For this review, take the finished solid that the model builds, in its own axes (mm). Face numbers are marked on the shaded views. A direction names the side the tool comes from. Coordinates: 2 decimals unless noted, no trailing zeros. Loops run counter-clockwise (first coordinate to the right, second up) from the corner with the lowest first, then second, coordinate; pieces in that order, holes last. Notation, with made-up numbers: (-24.75, 16.5) -> (-1.75, 16.5) arc R25 cw to (-1.75, 40.5) -> close; hole circle Ø9 at (40, 59). An arc over 180 degrees is marked (long way). Use a Markdown table: item, result.
from build123d import *

# Parameters (mm, degrees)
F0_W     = 38.1
F0_H     = 38.1
F1_DEPTH = 9.525
F2_SIZE  = 6.35
F3_W     = 38.1
F3_H     = 12.7
F4_DEPTH = 3.175


# Not quite as in the source:
# - a feature of the source that left no trace in its solid (it failed there, or was rolled back) is left out


with BuildPart() as f1:
    # F0 (on Top) → F1 (new body)
    with BuildSketch(Plane.XY):
        Rectangle(F0_W, F0_H)
    extrude(amount=F1_DEPTH)

    # F2
    f2_edges = [f1.edges().sort_by_distance(p)[0] for p in [
        (0, -19.05, 9.525),
    ]]
    chamfer(f2_edges, length=F2_SIZE)

    # F3 (on face) → F4 (join)
    with BuildSketch(Plane(origin=(0, 0, 0), x_dir=(1, 0, 0), z_dir=(0, 0, -1))):
        with Locations((0, 12.7)):
            Rectangle(F3_W, F3_H)
    extrude(amount=F4_DEPTH)


solid = f1.part
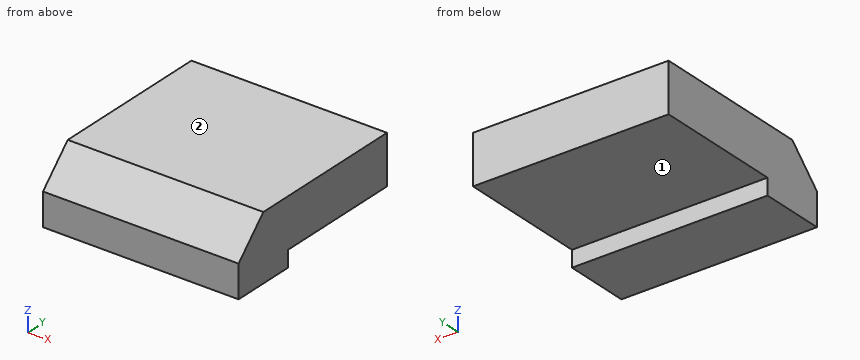
(1) Take a section at A-A on x = -15. Write out the cut boundary in (y, z) (3 decimals), plus the area to 3 significant figures.
Found:
| item | result |
|---|---|
| outline | (-19.05, -3.175) -> (-6.35, -3.175) -> (-6.35, 0) -> (19.05, 0) -> (19.05, 9.525) -> (-12.7, 9.525) -> (-19.05, 3.175) -> close |
| area | 383 mm^2 |
(2) For line 1 along Y through (x, z) = (-3, -1.5); line 2 along Z through (x, y) = (-7, -1) (3 decimals); line 3 along Y through (x, z) = (-12, 7.5) (3 decimals), list the stretches that pass through material, from the lowest coordinate up.
Found:
| item | result |
|---|---|
| line 1 | y = -19.05 to -6.35 |
| line 2 | z = 0 to 9.525 |
| line 3 | y = -14.725 to 19.05 |
(3) Take a section at B-B on y = 0.5. Write out the cut boundary in (x, z) (3 decimals).
Found:
| item | result |
|---|---|
| outline | (-19.05, 0) -> (19.05, 0) -> (19.05, 9.525) -> (-19.05, 9.525) -> close |
(4) For the marked faces 1 and 2, list the 3-axis set-ups (+Z, -Z, +X, -X, +Y, -Y) from which the entire face can be reached by the end or side of a thin tool; tool diameter is ignored.
Found:
| item | result |
|---|---|
| face 1 | -Z, +X, -X, +Y |
| face 2 | +Z, +X, -X, +Y, -Y |
(5) Take a section at C-C on z = 6.75. Write out the cut boundary in (x, y) (3 decimals).
Found:
| item | result |
|---|---|
| outline | (-19.05, -15.475) -> (19.05, -15.475) -> (19.05, 19.05) -> (-19.05, 19.05) -> close |
(6) For pin 1 Ø1 at (x, z) = (-1.5, -1) entering from +Y; pin 2 Ø6 at (x, y) = (-0.5, 11.5) entering from -Z, all flat-tipped, find the tip position at first contact; note any pin that passes through.
Found:
| item | result |
|---|---|
| pin 1 | stops at y = -6.35 |
| pin 2 | stops at z = 0 |
